Drawing for the job (mm, zero at the part's lowest x, y, z). Round coordinates to 2 decimals unless told otherwise and drop trailing zeros. Loops run counter-clockwise (first coordinate to the right, second up) from the corner with the lowest first, then second, coordinate; pieces in that order, holes last. Notation, with made-up numbers: M -13,17 L 18,17 A17 cw 18,42 Z; hole C 19.5,-13 d11. An arc over 180 degrees is marked long. Use a Markdown table: item, result. Add a question column.
Q1. Mould opens along Y. For the marked faces 1, 2 and 3 say: +Y half, -Y half, draft (parallel to the pull), parting line (faces both ways), or undercut.
Q2. Cut at C-C (z = 6). State how many separate pieces and enclosed holes the cut face has, plus the area to 3 significant figures.
Q3. Pin check, flat tips, straight feed: pin 1 (3 mm diameter, centred on y = 9.5, z = 5, fed in from -X); pin 2 (4 mm diameter, centred on x = 13.5, y = 31, fed in from +Z). Stop position of each tip, or through.
Q4. Cut at B-B (y = 29.75). Give the cut face in (x, z), plus the area to 3 significant figures.
Q5. Cut at D-D (x = 11.5). Give the cut face in (y, z).
Q6. Probe line 1 (Y direction, x = 37.5, z = 2.5); line 2 (X direction, y = 29.5, z = 2.25) (1 decimal); line 3 (Y direction, x = 17.5, z = 0.5) (1 decimal). List the from-to ranges inside material, lowest first. Write a range as from..to.
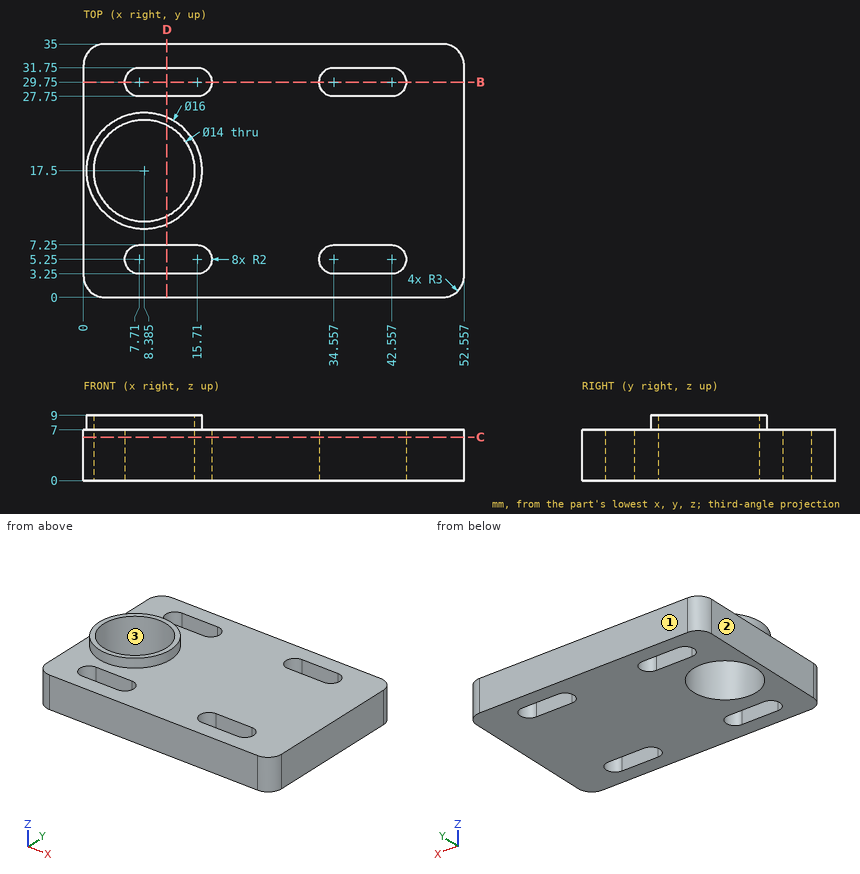
Checked values:
| question | item | result |
|---|---|---|
| 1 | face 1 | +Y half |
| 1 | face 2 | draft |
| 1 | face 3 | undercut |
| 2 | separate pieces | 1 |
| 2 | enclosed holes | 5 |
| 2 | area | 1,500 mm^2 |
| 3 | pin 1 | stops at x = 0 |
| 3 | pin 2 | stops at z = 7 |
| 4 | outline | M 0,0 L 5.71,0 L 5.71,7 L 0,7 Z; M 17.71,0 L 32.56,0 L 32.56,7 L 17.71,7 Z; M 44.56,0 L 52.56,0 L 52.56,7 L 44.56,7 Z |
| 4 | area | 200 mm^2 |
| 5 | outline | M 0,0 L 3.25,0 L 3.25,7 L 0,7 Z; M 7.25,0 L 11.23,0 L 11.23,9 L 10.13,9 L 10.13,7 L 7.25,7 Z; M 23.77,0 L 27.75,0 L 27.75,7 L 24.87,7 L 24.87,9 L 23.77,9 Z; M 31.75,0 L 35,0 L 35,7 L 31.75,7 Z |
| 6 | line 1 | y = 0..3.25, 7.25..27.75, 31.75..35 |
| 6 | line 2 | x = 0..5.7, 17.7..32.6, 44.5..52.6 |
| 6 | line 3 | y = 0..4.4, 6.1..28.9, 30.6..35 |
